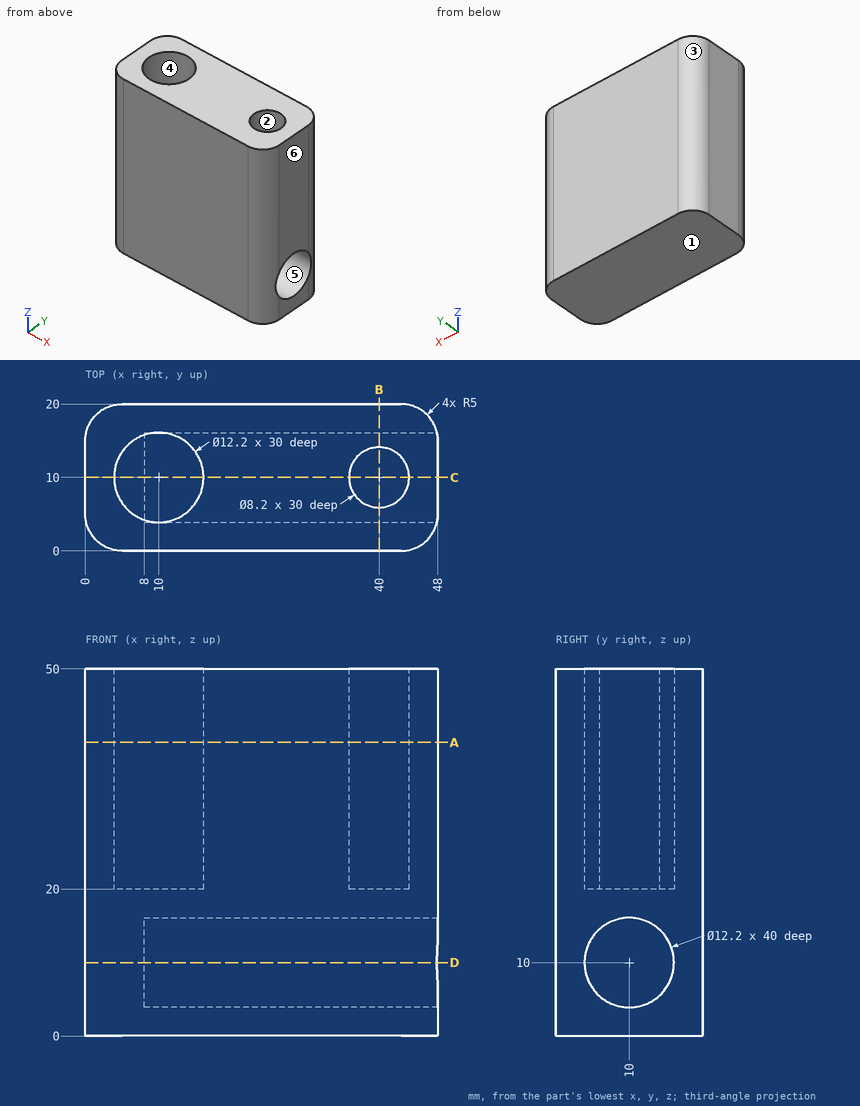
Source: three-view drawing plus pictorial views. Frame: mm from the lowest corner of the part. A direction names the side the tool comes from. Round coordinates to 2 decimals unless told otherwise and drop trailing zeros. Write each loop counter-clockwise with the first axis right and the second up, starting at its lowest first coordinate (ties: lowest second). Pieces come first, ordered by that corner, then holes. Notation, with made-up numbers: M 62.5,29 L 85.5,29 A17 cw 85.5,50 Z; hole C -32,73 d2. An arc over 180 degrees is marked long. One line per item, written item: value. Start each with the question number.
Item 1: Section query B-B (x = 40). Return the cut outline in (y, z).
Item 2: Mould query, pull axis X, two halves, no side actions, for the marked faces 1, 2 and 3. Classes: pulls with the +X half, pulls with the -X half, needs draft (parallel to the pull), parting line crosses it, or undercut.
Item 3: Section query D-D (z = 10). Return the cut outline in (x, y).
Item 4: Set-up query: the marked faces 4, 5 and 6. Return all of +Z, -Z, +X, -X, +Y, -Y with unobstructed straight access to the full face (end or side cutting, diameter ignored); none if empty.
Item 5: Pin query (flat end, axial travel): pin 1 (9 mm diameter, centred on x = 39, y = 9.5, fed in from +Z). Return the tip coordinate at first contact, or that it passes through.
Item 6: Ray query, L1, parallel to Y at x = 40, z = 42; L2, parallel to Y at x = 10, z = 33; L3, parallel to Z at x = 26, y = 13.5. Return the intervals inside material, ascending. Write a range as from..to.
Item 7: Section query C-C (y = 10). Return the cut outline in (x, z).
Item 8: Section query A-A (z = 40). Return the cut outline in (x, y), plus the area to 3 significant figures.
Result set:
1. outline: M 0,0 L 20,0 L 20,50 L 14.1,50 L 14.1,20 L 5.9,20 L 5.9,50 L 0,50 Z; hole C 10,10 d12.2
2. face 1: needs draft
2. face 2: undercut
2. face 3: pulls with the -X half
3. outline: M 0,5 A5 ccw 5,0 L 43,0 A5 ccw 47.88,3.9 L 8,3.9 L 8,16.1 L 47.88,16.1 A5 ccw 43,20 L 5,20 A5 ccw 0,15 Z
4. face 4: +Z
4. face 5: +X
4. face 6: +Z, -Z, +X, +Y, -Y
5. pin 1: stops at z = 50
6. L1: y = 0..5.9, 14.1..20
6. L2: y = 0..3.9, 16.1..20
6. L3: z = 0..5, 15..50
7. outline: M 0,0 L 48,0 L 48,3.9 L 8,3.9 L 8,16.1 L 48,16.1 L 48,50 L 44.1,50 L 44.1,20 L 35.9,20 L 35.9,50 L 16.1,50 L 16.1,20 L 3.9,20 L 3.9,50 L 0,50 Z
8. outline: M 0,5 A5 ccw 5,0 L 43,0 A5 ccw 48,5 L 48,15 A5 ccw 43,20 L 5,20 A5 ccw 0,15 Z; hole C 10,10 d12.2; hole C 40,10 d8.2
8. area: 769 mm²
